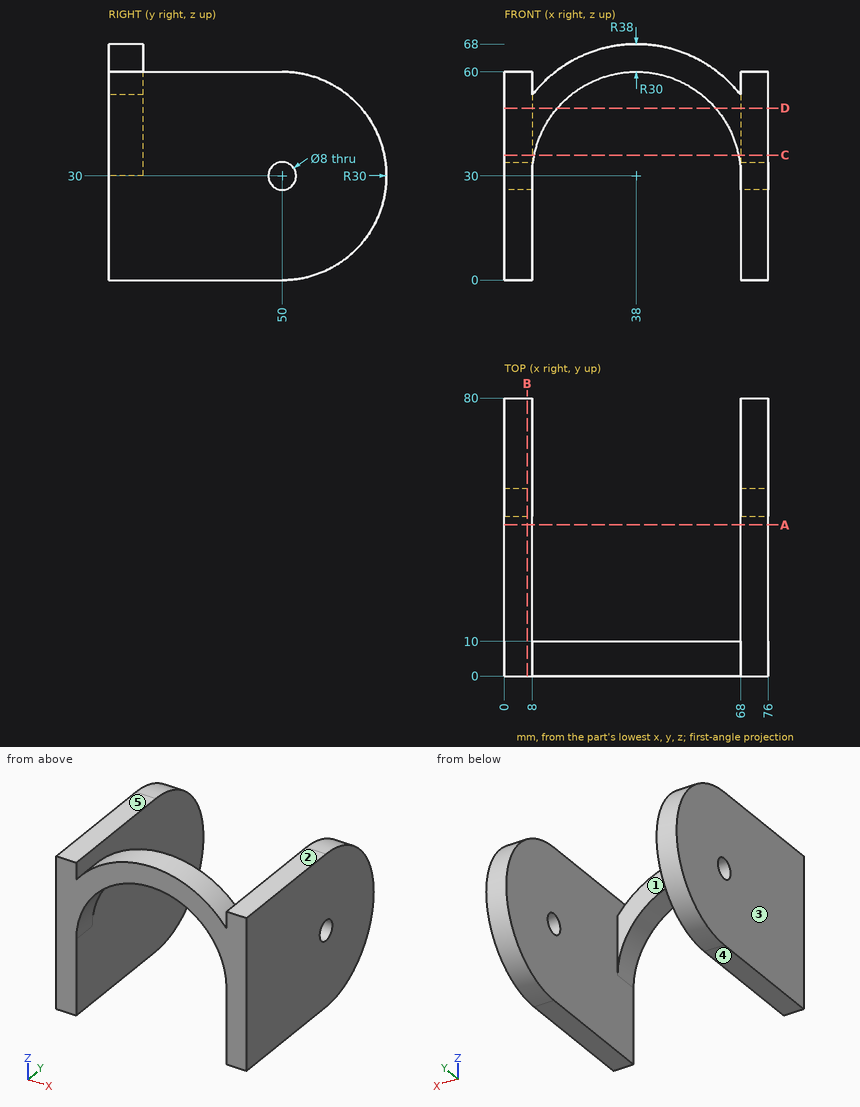
Answer from the drawing. Dimensions are ordinates in mm from the lowest x, y and z of the part. A direction names the side the tool comes from. Coordinates: 2 decimals unless noted, no trailing zeros. Loops run counter-clockwise (first coordinate to the right, second up) from the corner with the lowest first, then second, coordinate; pieces in that order, holes last.
1) For the marked faces 4 and 5, determine the directions among +Z, -Z, +X, -X, +Y, -Y from which every point of the face is accessible in a straight line to the end or side of a thin tool.
Results:
face 4: -Z, +X, -X, +Y, -Y
face 5: +Z, -X, +Y, -Y
2) For a pull along X with two mould halves and no side action, classify the marked faces 1, 2 and 3 as +X half, -X half, draft (parallel to the pull), parting line (faces both ways), or undercut.
Results:
face 1: undercut
face 2: draft
face 3: -X half
3) Section B-B (x = 6.5) is taken. Give the vertices of the cut face in (y, z).
Results:
outline: (0, 0) - (50, 0) arc R30 ccw to (50, 60) - (0, 60) - close; hole circle Ø8 at (50, 30)
4) Flat-ended cylindrical pins translate along their axes: pin 1 (9 mm diameter, centred on x = 70.5, y = 17.5, fed in from +Z); pin 2 (8 mm diameter, centred on x = 19.5, z = 44.5, fed in from -Y); pin 3 (3 mm diameter, centred on x = 34, y = 10.5, fed in from -Z). Find the tip coordinate at first contact, or state that the pin passes through.
Results:
pin 1: stops at z = 60
pin 2: passes through
pin 3: stops at z = 59.51
5) Section A-A (y = 43.5) is taken. Give the vertices of the cut face in (x, z), plus the area to 3 significant figures.
Results:
outline: (0, 0) - (8, 0) - (8, 60) - (0, 60) - close; (68, 0) - (76, 0) - (76, 60) - (68, 60) - close
area: 960 mm2
6) Section C-C (z = 36) is taken. Give the vertices of the cut face in (x, y), plus the area to 3 significant figures.
Results:
outline: (0, 0) - (8.61, 0) - (8.61, 10) - (8, 10) - (8, 79.39) - (0, 79.39) - close; (67.39, 0) - (76, 0) - (76, 79.39) - (68, 79.39) - (68, 10) - (67.39, 10) - close
area: 1,280 mm2
7) Consider probe 1 along Y at (x, z) = (71.75, 30); probe 2 along X at (y, z) = (60, 35); probe 3 along Z at (x, y) = (71, 33). Determine where each line is inside the solid, lowest interval first.
Results:
probe 1: y = 0 to 46, 54 to 80
probe 2: x = 0 to 8, 68 to 76
probe 3: z = 0 to 60
8) Section D-D (z = 49.5) is taken. Give the vertices of the cut face in (x, y), plus the area to 3 significant figures.
Results:
outline: (0, 0) - (15.2, 0) - (15.2, 10) - (8, 10) - (8, 72.8) - (0, 72.8) - close; (60.8, 0) - (76, 0) - (76, 72.8) - (68, 72.8) - (68, 10) - (60.8, 10) - close
area: 1,310 mm2
